Input: dimensioned drawing with shaded views. Units: mm. Origin: part minimum x, y, z. A direction names the side the tool comes from. Give positions to 0.01 mm unless a question says otherwise; leave off trailing zeros. Write each loop counter-clockwise with the first axis right and the second up, starting at its lowest first coordinate (ties: lowest second). Pieces come first, ordered by that corner, then holes. Notation, with made-up numbers: (33, 87) -> (80, 87) arc R26 cw to (80, 111) -> close; hole circle Ø8 at (52, -24.5). An arc over 180 degrees is marked (long way). Answer as a JSON object with one key per item and string values.
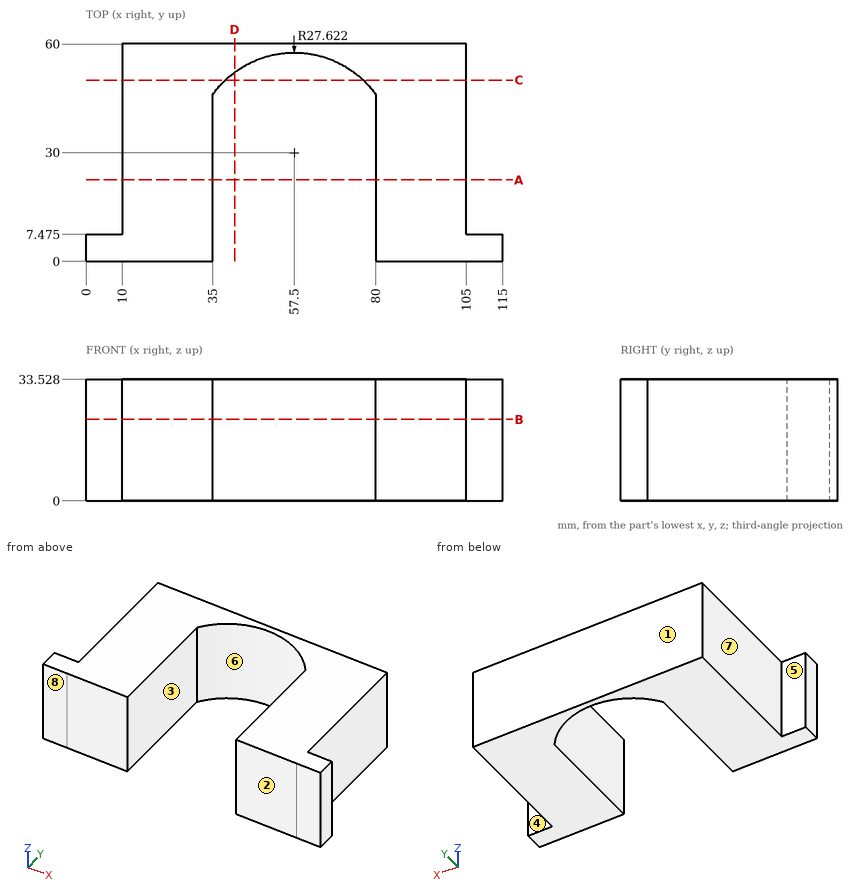
Q1. Cut plane D-D (x = 41). Return the cut outline in (y, z), and give its area (3 significant figures).
Values:
{"outline": "(52.15, 0) -> (60, 0) -> (60, 33.53) -> (52.15, 33.53) -> close", "area": "263 mm²"}
Q2. Cut plane C-C (y = 50). Return the cut outline in (x, z).
Values:
{"outline": "(10, 0) -> (38.45, 0) -> (38.45, 33.53) -> (10, 33.53) -> close; (76.55, 0) -> (105, 0) -> (105, 33.53) -> (76.55, 33.53) -> close"}
Q3. First-contact query: P1, Ø5, axis at y = 26, z = 20.5, coming from the +X side; P2, Ø3, axis at y = 44, z = 9.5, coming from the -X side. Flat tips, straight axial feed; report the tip coordinate or a pass-through.
Values:
{"P1": "x = 105", "P2": "x = 10"}
Q4. Cut plane A-A (y = 22.5). Return the cut outline in (x, z), and give its area (3 significant figures).
Values:
{"outline": "(10, 0) -> (35, 0) -> (35, 33.53) -> (10, 33.53) -> close; (80, 0) -> (105, 0) -> (105, 33.53) -> (80, 33.53) -> close", "area": "1,680 mm²"}
Q5. Cut plane B-B (z = 22.5). Return the cut outline in (x, y) (1 decimal), and give its area (3 significant figures).
Values:
{"outline": "(0, 0) -> (35, 0) -> (35, 46) arc R27.6 cw to (80, 46) -> (80, 0) -> (115, 0) -> (115, 7.5) -> (105, 7.5) -> (105, 60) -> (10, 60) -> (10, 7.5) -> (0, 7.5) -> close", "area": "3,410 mm²"}
Q6. Material intervals for L1, parallel to X at y = 42, z = 13.5; L2, parallel to X at y = 3, z = 14; L3, parallel to Y at x = 58, z = 7, sorted ascending. Write a range as from..to.
Values:
{"L1": "10..35, 80..105", "L2": "0..35, 80..115", "L3": "57.62..60"}
Q7. Set-up query: the marked faces 1, 2, 3, 4 and 5. Return all of +Z, -Z, +X, -X, +Y, -Y with unobstructed straight access to the full face (end or side cutting, diameter ignored); none if empty.
Values:
{"face 1": "+Z, -Z, +X, -X, +Y", "face 2": "+Z, -Z, +X, -X, -Y", "face 3": "+Z, -Z, -Y", "face 4": "+Z, -Z, +X, +Y", "face 5": "+Z, -Z, -X, +Y"}
Q8. Mould query, pull axis X, two halves, no side actions, for the marked faces 6, 7 and 8. Classes: pulls with the +X half, pulls with the -X half, needs draft (parallel to the pull), parting line crosses it, or undercut.
Values:
{"face 6": "undercut", "face 7": "pulls with the -X half", "face 8": "needs draft"}
